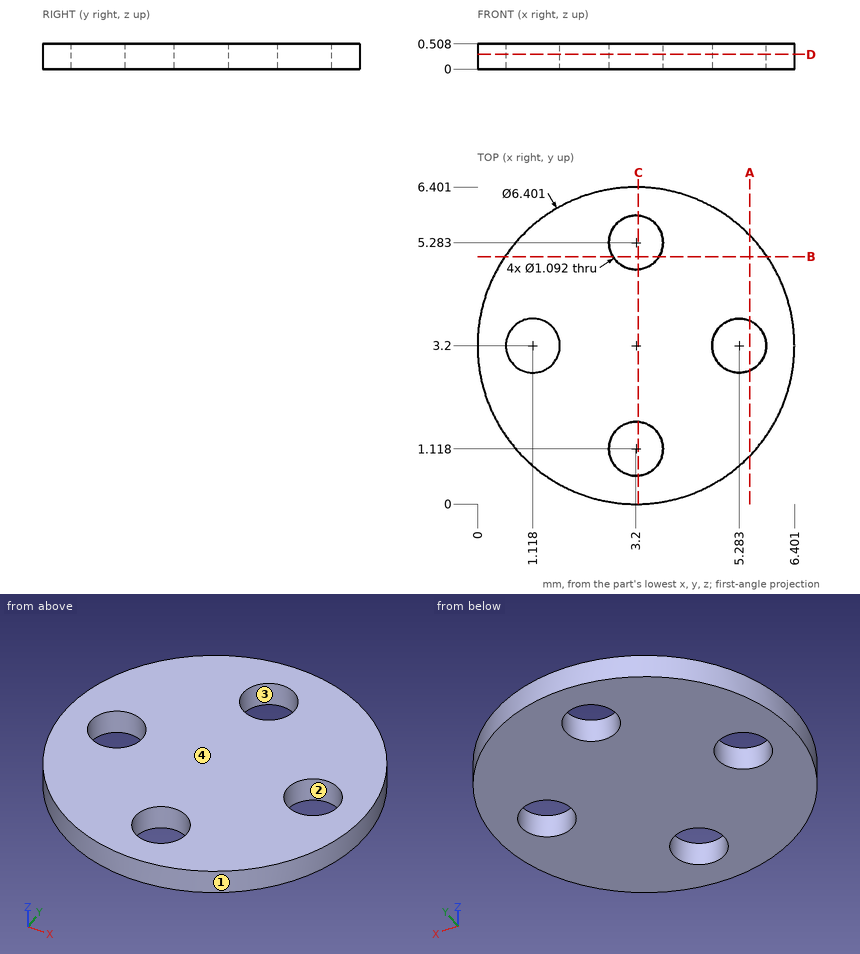
Print and shaded views of the part. All mm, measured from the part's lowest x, y and z. Give positions to 0.01 mm unless a question says otherwise; leave off trailing zeros. Order: outer loops, then holes, each group sorted by start corner. A loop starts at its lowest first (then second) coordinate and runs counter-clockwise, first axis right, second up. Notation, with made-up numbers: (38, 37) -> (63, 37) arc R18 cw to (63, 53) -> close; hole circle Ø7 at (73.5, -36). An arc over 180 degrees is marked (long way). Use CSV: the item, a comma, the result in double quotes.
1. Drop a flat-ended pin along its axis: pin 1 (1.7 mm diameter, centred on x = 3.2, y = 1.12, fed in from +Z). Give the stop position or say it passes through.
Outcome:
pin 1,"z = 0.51"
2. Band-saw the part on A-A, the plane x = 5.5. Give the cut face in (y, z) (1 decimal).
Outcome:
outline,"(1, 0) -> (2.7, 0) -> (2.7, 0.5) -> (1, 0.5) -> close; (3.7, 0) -> (5.4, 0) -> (5.4, 0.5) -> (3.7, 0.5) -> close"
3. Mould opens along X. For the marked faces 1, 2, 3 and 4 say: +X half, -X half, draft (parallel to the pull), parting line (faces both ways), or undercut.
Outcome:
face 1,"parting line"
face 2,"undercut"
face 3,"undercut"
face 4,"draft"
4. Band-saw the part on C-C, the plane x = 3.25. Give the cut face in (y, z).
Outcome:
outline,"(0, 0) -> (0.57, 0) -> (0.57, 0.51) -> (0, 0.51) -> close; (1.66, 0) -> (4.74, 0) -> (4.74, 0.51) -> (1.66, 0.51) -> close; (5.83, 0) -> (6.4, 0) -> (6.4, 0.51) -> (5.83, 0.51) -> close"
5. Band-saw the part on B-B, the plane y = 5. Give the cut face in (x, z).
Outcome:
outline,"(0.55, 0) -> (2.73, 0) -> (2.73, 0.51) -> (0.55, 0.51) -> close; (3.67, 0) -> (5.85, 0) -> (5.85, 0.51) -> (3.67, 0.51) -> close"
6. Drill centre lines: line 1 along Y through (x, z) = (3.5, 0.3) (1 decimal); line 2 along X through (y, z) = (3, 0.4) (1 decimal); line 3 along X through (y, z) = (2.75, 0.1) (1 decimal). Where is each one in solid material? Low to high. Write a range as from..to.
Outcome:
line 1,"0..0.7, 1.6..4.8, 5.7..6.4"
line 2,"0..0.6, 1.6..4.8, 5.8..6.4"
line 3,"0..0.8, 1.4..5, 5.6..6.4"
7. Band-saw the part on D-D, the plane z = 0.3. Give the cut face in (x, y).
Outcome:
outline,"circle Ø6.4 at (3.2, 3.2); hole circle Ø1.09 at (1.12, 3.2); hole circle Ø1.09 at (3.2, 1.12); hole circle Ø1.09 at (3.2, 5.28); hole circle Ø1.09 at (5.28, 3.2)"
